```python
from build123d import *

# Parameters (mm, degrees)
ESQUISSE1_W        = 66
ESQUISSE1_H        = 43.5
BOSS_EXTRU_1_DEPTH = 22
ESQUISSE2_W        = 51
ESQUISSE2_H        = 43.5
BOSS_EXTRU_2_DEPTH = 8
ESQUISSE3_W        = 11.5
ESQUISSE3_H        = 7.5
ESQUISSE3_W_2      = 6
ESQUISSE3_H_2      = 4
BOSS_EXTRU_3_DEPTH = 2.5
CONG_1_R           = 2


with BuildPart() as part:
    # Esquisse1 → Boss.-Extru.1 (new body)
    with BuildSketch(Plane.XY):
        with Locations((2.845632419, 0)):
            Rectangle(ESQUISSE1_W, ESQUISSE1_H)
    extrude(amount=BOSS_EXTRU_1_DEPTH)

    # Esquisse2 → Boss.-Extru.2 (add)
    with BuildSketch(Plane.XY.offset(22)):
        with Locations((10.345632419, 0)):
            Rectangle(ESQUISSE2_W, ESQUISSE2_H)
    extrude(amount=BOSS_EXTRU_2_DEPTH)

    # Esquisse3 → Boss.-Extru.3 (add)
    # profile 1 of 2: a face of its own
    with BuildSketch(Plane(origin=(0, 0, 0), x_dir=(-1, 0, 0), z_dir=(0, 0, -1))):
        with Locations((-9.595632419, 25.5)):
            Rectangle(ESQUISSE3_W, ESQUISSE3_H)
        with Locations((-9.595632419, 24.95)):
            Rectangle(ESQUISSE3_W_2, ESQUISSE3_H_2, mode=Mode.SUBTRACT)
    # profile 2 of 2: a face of its own
    with BuildSketch(Plane(origin=(0, 0, 0), x_dir=(-1, 0, 0), z_dir=(0, 0, -1))):
        with Locations((-9.595632419, -25.5)):
            Rectangle(ESQUISSE3_W, ESQUISSE3_H)
        with Locations((-9.595632419, -24.95)):
            Rectangle(ESQUISSE3_W_2, ESQUISSE3_H_2, mode=Mode.SUBTRACT)
    extrude(amount=-BOSS_EXTRU_3_DEPTH)

    # Congé1
    cong_1_edges = [part.edges().sort_by_distance(p)[0] for p in [
        (-15.154367581, 21.75, 26),
        (-15.154367581, -21.75, 26),
        (10.345632419, -21.75, 30),
        (35.845632419, 0, 30),
        (10.345632419, 21.75, 30),
        (-15.154367581, 0, 30),
        (15.345632419, 29.25, 1.25),
        (3.845632419, 29.25, 1.25),
        (-30.154367581, 0, 22),
        (15.345632419, -29.25, 1.25),
        (3.845632419, -29.25, 1.25),
        (35.845632419, 21.75, 15),
        (35.845632419, -21.75, 15),
    ]]
    fillet(cong_1_edges, radius=CONG_1_R)


solid = part.part
```
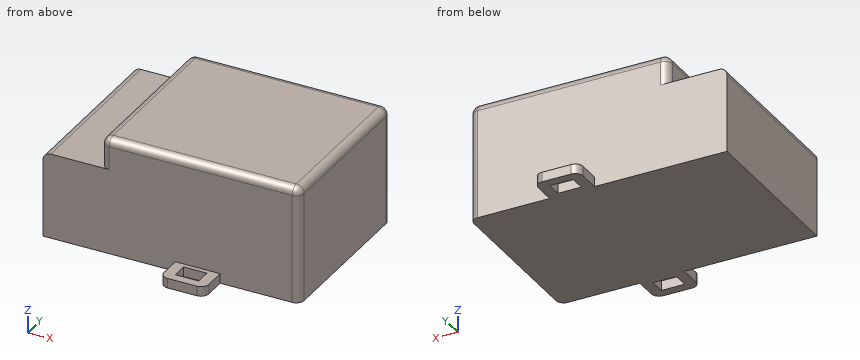
The listing builds one solid part. Answer for the finished solid, in the listing's coordinates (mm). Round coordinates to 2 decimals unless told otherwise and drop trailing zeros. Order: outer loops, then holes, each group sorted by start corner. A loop starts at its lowest first (then second) coordinate and runs counter-clockwise, first axis right, second up. Notation, with made-up numbers: (47.25, 17.25) - (75.25, 17.25) arc R26 cw to (75.25, 55.25) - close; hole circle Ø7 at (7, 0). An arc over 180 degrees is marked (long way). Put each result on its own line as item: value. Start each with the question number.
(1) Find section C-C (z = 24.75). Give the vertices of the cut face in (x, y), plus the area to 3 significant figures.
(2) Find section A-A (x = 10.5). Give the vertices of the cut face in (y, z).
(3) Straight lines are drawn through the part: probe 1 along X at (y, z) = (-4.5, 27.5); probe 2 along Z at (x, y) = (-23, -6); probe 3 along Y at (x, z) = (22, 18). For each, find the intervals that lie inside material, in ascending order. Write a range as from..to.
(4) Find section B-B (y = -25). Give the vertices of the cut face in (x, z), plus the area to 4 significant figures.
(5) Given P1, Ø3, axis at x = 0.5, z = 24, coming from the +Y side; P2, Ø0.8, axis at y = 23.5, z = 0.5, coming from the +X side; P3, Ø1.2, axis at y = 25.5, z = 1.5, coming from the -X side, each flat-ended and moving along its own axis, determine where each tip first touches the part or whether it passes through.
(6) Find section D-D (y = -3). Give the vertices of the cut face in (x, z), plus the area to 3 significant figures.
Reply:
1. outline: (-15.15, -19.75) arc R2 ccw to (-13.15, -21.75) - (33.85, -21.75) arc R2 ccw to (35.85, -19.75) - (35.85, 19.75) arc R2 ccw to (33.85, 21.75) - (-13.15, 21.75) arc R2 ccw to (-15.15, 19.75) - close
1. area: 2,220 mm^2
2. outline: (-29.25, 0) - (-26.95, 0) - (-26.95, 2.5) - (-29.25, 2.5) - close; (-22.95, 0) - (22.95, 0) - (22.95, 2.5) - (21.75, 2.5) - (21.75, 28) arc R2 ccw to (19.75, 30) - (-19.75, 30) arc R2 ccw to (-21.75, 28) - (-21.75, 2.5) - (-22.95, 2.5) - close; (26.95, 0) - (29.25, 0) - (29.25, 2.5) - (26.95, 2.5) - close
3. probe 1: -15.15..35.85
3. probe 2: 0..22
3. probe 3: -21.75..21.75
4. outline: (3.85, 0) - (6.6, 0) - (6.6, 2.5) - (3.85, 2.5) - close; (12.6, 0) - (15.35, 0) - (15.35, 2.5) - (12.6, 2.5) - close
4. area: 13.75 mm^2
5. P1: y = 21.75
5. P2: x = 15.35
5. P3: x = 3.85
6. outline: (-30.15, 0) - (35.85, 0) - (35.85, 28) arc R2 ccw to (33.85, 30) - (-13.15, 30) arc R2 ccw to (-15.15, 28) - (-15.15, 22) - (-28.15, 22) arc R2 ccw to (-30.15, 20) - close
6. area: 1,860 mm^2
